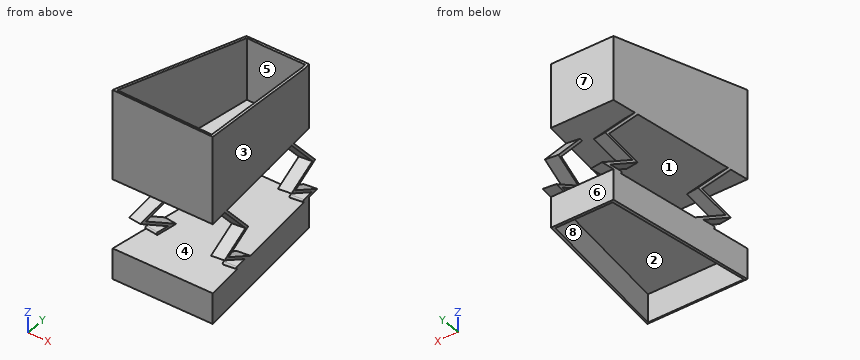
from build123d import *

# Parameters (mm, degrees)
BOSS_EXTRUDE1_DEPTH = 350
SHELL1_T            = -10
CUT_EXTRUDE1_DEPTH  = 436
SKETCH3_W           = 259.761046689
SKETCH3_H           = 96.41009556
CUT_EXTRUDE2_DEPTH  = 653.147409369
BOSS_EXTRUDE2_DEPTH = 50
BOSS_EXTRUDE3_DEPTH = 120
CUT_EXTRUDE3_DEPTH  = 110


with BuildPart() as part:
    # Sketch1 → Boss-Extrude1 (new body)
    with BuildSketch(Plane.XY):
        Polygon((-125, 424.335548173), (125, 424.335548173), (200, -175.664451827), (-200, -175.664451827), align=None)
    extrude(amount=BOSS_EXTRUDE1_DEPTH)

    # Shell1
    shell1_openings = [part.faces().sort_by_distance(p)[0] for p in [
        (0, 101.258625096, 350),
    ]]
    offset(amount=SHELL1_T, openings=shell1_openings, kind=Kind.INTERSECTION)

    # Sketch2 → Cut-Extrude1 (cut)
    with BuildSketch(Plane(origin=(-175.302836698, 21.912854587, 0), x_dir=(0, 0, 1), z_dir=(-0.9922778767136677, 0.12403473458920852, 0))):
        Polygon((250, 405.554434931), (350, -199.114896191), (350, 405.554434931), align=None)
    extrude(amount=-CUT_EXTRUDE1_DEPTH, mode=Mode.SUBTRACT)

    # Sketch3 → Cut-Extrude2 (cut, through all)
    with BuildSketch(Plane(origin=(-175.302836698, 21.912854587, 0), x_dir=(0, 0, 1), z_dir=(-0.9922778767136677, 0.12403473458920852, 0))):
        with Locations((379.880523345, 453.759482711)):
            Rectangle(SKETCH3_W, SKETCH3_H)
    extrude(amount=-CUT_EXTRUDE2_DEPTH, mode=Mode.SUBTRACT)

    # Sketch5 → Boss-Extrude2 (add)
    with BuildSketch(Plane(origin=(-175.302836698, 21.912854587, 0), x_dir=(0, 0, 1), z_dir=(-0.9922778767136677, 0.12403473458920852, 0))):
        with BuildLine():
            Line((0, -124.744929756), (-142.467162168, 5.816018008))
            Line((-142.467162168, 5.816018008), (-187.751575152, -124.744929756))
            Line((-187.751575152, -124.744929756), (-260.206635925, 0))
            Line((-260.206635925, 0), (-260.206635925, -46.209963839))
            ThreePointArc((-260.206635925, -46.209963839), (-265.206635925, -51.209963839), (-270.206635925, -46.209963839))
            Line((-270.206635925, -46.209963839), (-270.206635925, 37.127182563))
            Line((-270.206635925, 37.127182563), (-190.054813406, -100.869161145))
            Line((-190.054813406, -100.869161145), (-146.928792702, 23.468856407))
            Line((-146.928792702, 23.468856407), (6.756291537, -117.372513282))
            ThreePointArc((6.756291537, -117.372513282), (7.064354006, -124.436867288), (0, -124.744929756))
        make_face()
        with BuildLine():
            Line((0, 295.255070244), (-142.467162168, 425.816018008))
            Line((-142.467162168, 425.816018008), (-187.751575152, 295.255070244))
            Line((-187.751575152, 295.255070244), (-260.206635925, 420))
            Line((-260.206635925, 420), (-260.206635925, 373.790036161))
            ThreePointArc((-260.206635925, 373.790036161), (-265.206635925, 368.790036161), (-270.206635925, 373.790036161))
            Line((-270.206635925, 373.790036161), (-270.206635925, 457.127182563))
            Line((-270.206635925, 457.127182563), (-190.054813406, 319.130838855))
            Line((-190.054813406, 319.130838855), (-146.928792702, 443.468856407))
            Line((-146.928792702, 443.468856407), (6.756291537, 302.627486718))
            ThreePointArc((6.756291537, 302.627486718), (7.064354006, 295.563132712), (0, 295.255070244))
        make_face()
    boss_extrude2 = extrude(amount=-BOSS_EXTRUDE2_DEPTH)

    # Mirror1: Boss-Extrude2 across plane
    add(boss_extrude2.mirror(Plane(origin=(0, 0, 0), x_dir=(0, 0, 1), z_dir=(1, 0, 0))))

    # Sketch6 → Boss-Extrude3 (add)
    with BuildSketch(Plane(origin=(0, 0, -270.206635925), x_dir=(-1, 0, 0), z_dir=(0, 0, -1))):
        Polygon((-200, -175.664451827), (-125, 424.335548173), (125, 424.335548173), (200, -175.664451827), align=None)
    extrude(amount=BOSS_EXTRUDE3_DEPTH)

    # Sketch7 → Cut-Extrude3 (cut)
    with BuildSketch(Plane(origin=(0, 0, -390.206635925), x_dir=(-1, 0, 0), z_dir=(0, 0, -1))):
        Polygon((-192.972753686, -170.052955611), (-114.88610452, 414.250591596), (113.988556829, 414.250591596), (190.280110611, -170.052955611), align=None)
    extrude(amount=-CUT_EXTRUDE3_DEPTH, mode=Mode.SUBTRACT)


solid = part.part
CAD build for the part. Positions are in the model's coordinates, mm. Face numbers are marked on the shaded views. A direction names the side the tool comes from. Round coordinates to 2 decimals unless told otherwise and drop trailing zeros. Loops run counter-clockwise (first coordinate to the right, second up) from the corner with the lowest first, then second, coordinate; pieces in that order, holes last.
(1) Cut at B-B (x = -31.5). Give the cut face in (y, z), plus the area to 3 significant figures.
(2) Which spindle directions (+Z, -Z, +X, -X, +Y, -Y) get a long thin tool onto all of the face, cutting with end or side? Do the marked faces 5, 6, 7 and 8. Say none if no direction does.
(3) Drop flat-ended pins along their axis: pin 1 (10 mm diameter, centred on x = 153.5, y = -69.5, fed in from -Z); pin 2 (10 mm diameter, centred on x = 86.5, y = -58, fed in from +Z); pin 3 (3 mm diameter, centred on y = -98.5, z = 69, fed in from -X). Give the stop position or say it passes through.
(4) Two-plate mould, pull along Z, no slides. Class the marked faces 1, 2, 3 and 4: +Z half, -Z half, draft (parallel to the pull), parting line (faces both ways), or undercut.
(5) Cut at A-A (z = 99). Give the cut face in (x, y), plus the area to 3 significant figures.
(6) Cut at D-D (z = -321.5). Give the cut face in (x, y), plus the area to 3 significant figures.
(7) Wall check: line 1 along Z through (x, y) = (-94, 25); line 2 along Y through (x, z) = (-11.5, -333); line 3 along X through (y, z) = (-4, 35.5). Give the ranges that are in metal, low to high.
(8) Cut at C-C (y = 173.5). Give the cut face in (x, z), plus the area to 3 significant figures.
Findings below:
1. outline: (-175.66, -390.21) - (-170.05, -390.21) - (-170.05, -280.21) - (414.25, -280.21) - (414.25, -390.21) - (424.34, -390.21) - (424.34, -270.21) - (-175.66, -270.21) - close; (-175.66, 0) - (424.34, 0) - (424.34, 250) - (414.34, 250) - (414.34, 10) - (-165.66, 10) - (-165.66, 344.9) - (-175.66, 346.54) - close
1. area: 19,500 mm2
2. face 5: +Z
2. face 6: -Z, +X, -X, +Y
2. face 7: +Z, +X, -X, +Y
2. face 8: -Z
3. pin 1: stops at z = -280.21
3. pin 2: stops at z = 10
3. pin 3: stops at x = -190.54
4. face 1: undercut
4. face 2: -Z half
4. face 3: draft
4. face 4: undercut
5. outline: (-200, -175.66) - (200, -175.66) - (125, 424.34) - (-125, 424.34) - close; hole (-188.67, -165.66) - (188.67, -165.66) - (116.17, 414.34) - (-116.17, 414.34) - close
5. area: 18,200 mm2
6. outline: (-200, -175.66) - (200, -175.66) - (125, 424.34) - (-125, 424.34) - close; hole (-190.28, -170.05) - (192.97, -170.05) - (114.89, 414.25) - (-113.99, 414.25) - close
6. area: 16,200 mm2
7. line 1: z = -280.21 to -270.21, 0 to 10
7. line 2: y = -175.66 to -170.05, 414.25 to 424.34
7. line 3: x = -178.54 to -168.46, 168.46 to 178.54
8. outline: (-156.35, -390.21) - (-145.42, -390.21) - (-145.42, -280.21) - (147.06, -280.21) - (147.06, -390.21) - (156.35, -390.21) - (156.35, -270.21) - (-156.35, -270.21) - close; (-156.35, 0) - (156.35, 0) - (156.35, 285.39) - (146.28, 285.6) - (146.28, 10) - (-146.28, 10) - (-146.28, 291.6) - (-156.35, 291.81) - close
8. area: 14,100 mm2
